Autodesk Inventor part; units mm, degrees
ref_plane "YZ Plane" through (0, 0, 0) normal (1, 0, 0) x (0, 1, 0)
ref_plane "XZ Plane" through (0, 0, 0) normal (0, 1, 0) x (-1, 0, 0)
ref_plane "XY Plane" through (0, 0, 0) normal (0, 0, 1) x (1, 0, 0)
sketch "Sketch1" plane through (0, 0, 0) normal (1, 0, 0) x (0, 1, 0)
  line L0 (0, -1) -> (-5, -1)
  line L1 (-5, -1) -> (-5, 0)
  line L2 (-4.5, -3.5) -> (-6.8, -3.5)
  line L3 (-6, -1.5) -> (-13, -1.5)
  line L4 (-13, -1.5) -> (-13, 0)
  line L5 (-6, -1.5) -> (-6, -3)
  line L6 (-6, -3) -> (-6.8, -3)
  line L7 (-6.8, -3) -> (-6.8, -3.5)
  line L8 (0, 0) -> (-1.5156, 0)
  line L9 (-5, 0) -> (-13, 0)
  line L10 (0, -1) -> (0, -1.75)
  line L11 (0, -1.75) -> (-4.5, -1.75)
  line L12 (-4.5, -1.75) -> (-4.5, -3.5)
  dimension "d4" = 0.5
  dimension "d5" = 1.5
  dimension "d6" = 0.8
  dimension "d7" = 1
  dimension "d11" = 8
  dimension "d12" = 2
  dimension "d13" = 5
  dimension "d14" = 3
  dimension "d15" = 1.5
  dimension "d16" = 3.5
  dimension "d17" = 7
revolve "Revolution1" add sketch "Sketch1" angle 360 about axis through (0, 0, 0) along (0, -1, 0)
thread "Thread1"
properties part number "042"
The listing builds one solid part. Answer for the finished solid, in the listing's coordinates (mm). A direction names the side the tool comes from. Round coordinates to 2 decimals unless told otherwise and drop trailing zeros. Write each loop counter-clockwise with the first axis right and the second up, starting at its lowest first coordinate (ties: lowest second). Pieces come first, ordered by that corner, then holes. Notation, with made-up numbers: M 68.5,59 L 120.5,59 A30 ccw 120.5,81 Z; hole C 34.5,29.25 d7. An arc over 180 degrees is marked long. Write each question's results on one line, items separated by ' | '. Start each with the question number.
Item 1: Given pin 1 Ø2 at (y, z) = (-8, 1) entering from +X; pin 2 Ø1.5 at (x, y) = (0.5, -2.5) entering from +Z; pin 3 Ø1.5 at (x, y) = (2, -9.5) entering from -Z, each flat-ended and moving along its own axis, determine where each tip first touches the part or whether it passes through.
Item 2: Which of the six approach directions +Z, -Z, +X, -X, +Y, -Y give full straight-line access (tool end or side, diameter ignored) to faces 1 (the cylindrical face through (-1.341, -5.666, -3.233)), 2 (the flat face through (-1.3, -6, -1.3)), 3 (the flat face through (0, -5, 0))?
Item 3: Find section C-C on z = 2.5. Write down the section's boundary in (x, y).
Item 4: The mould has two halves that part along X. Classify faces 4 (the cylindrical face through (-1, -3, 0)), 5 (the cylindrical face through (-0.67, -2.282, -1.617)), 6 (the flat face through (-1, 0, -1)): +X half, -X half, draft (parallel to the pull), parting line (faces both ways), or undercut.
Item 5: Find section D-D on x = -1.25. Write down the section's boundary in (y, z), and give its area (3 significant figures).
Item 6: Straight lines are drawn through the part: probe 1 along X at (y, z) = (-3.05, 0); probe 2 along X at (y, z) = (-6.25, 0.5); probe 3 along Y at (x, z) = (2.25, 0). For each, find the intervals that lie inside material, in ascending order.
Item 7: Find section B-B on x = 0. Write down the section's boundary in (y, z), and give its area (4 significant figures).
Item 8: Find section A-A on y = -6.5. Write down the section's boundary in (x, z), and give its area (3 significant figures).
Answer block:
1) pin 1: stops at x = 1.5 | pin 2: stops at z = 1.75 | pin 3: stops at z = -0.83
2) face 1: +Y, -Y | face 2: -Y | face 3: +Y
3) outline: M -2.45,-6.8 L -1.66,-6.8 L -1.66,-6 L 1.66,-6 L 1.66,-6.8 L 2.45,-6.8 L 2.45,-4.5 L -2.45,-4.5 Z
4) face 4: undercut | face 5: parting line | face 6: draft
5) outline: M -13,-0.83 L -6,-0.83 L -6,-2.73 L -6.8,-2.73 L -6.8,-3.27 L -4.5,-3.27 L -4.5,-1.22 L 0,-1.22 L 0,1.22 L -4.5,1.22 L -4.5,3.27 L -6.8,3.27 L -6.8,2.73 L -6,2.73 L -6,0.83 L -13,0.83 Z | area: 33.3 mm²
6) probe 1: x = -1.75 to -1, 1 to 1.75 | probe 2: x = -3.46 to -2.96, -1.41 to 1.41, 2.96 to 3.46 | probe 3: y = -6 to -4.5
7) outline: M -13,-1.5 L -6,-1.5 L -6,-3 L -6.8,-3 L -6.8,-3.5 L -4.5,-3.5 L -4.5,-1.75 L 0,-1.75 L 0,-1 L -5,-1 L -5,1 L 0,1 L 0,1.75 L -4.5,1.75 L -4.5,3.5 L -6.8,3.5 L -6.8,3 L -6,3 L -6,1.5 L -13,1.5 Z | area: 38.05 mm²
8) outline: C 0,0 d7; C 0,0 d3; hole C 0,0 d6 | area: 17.3 mm²
